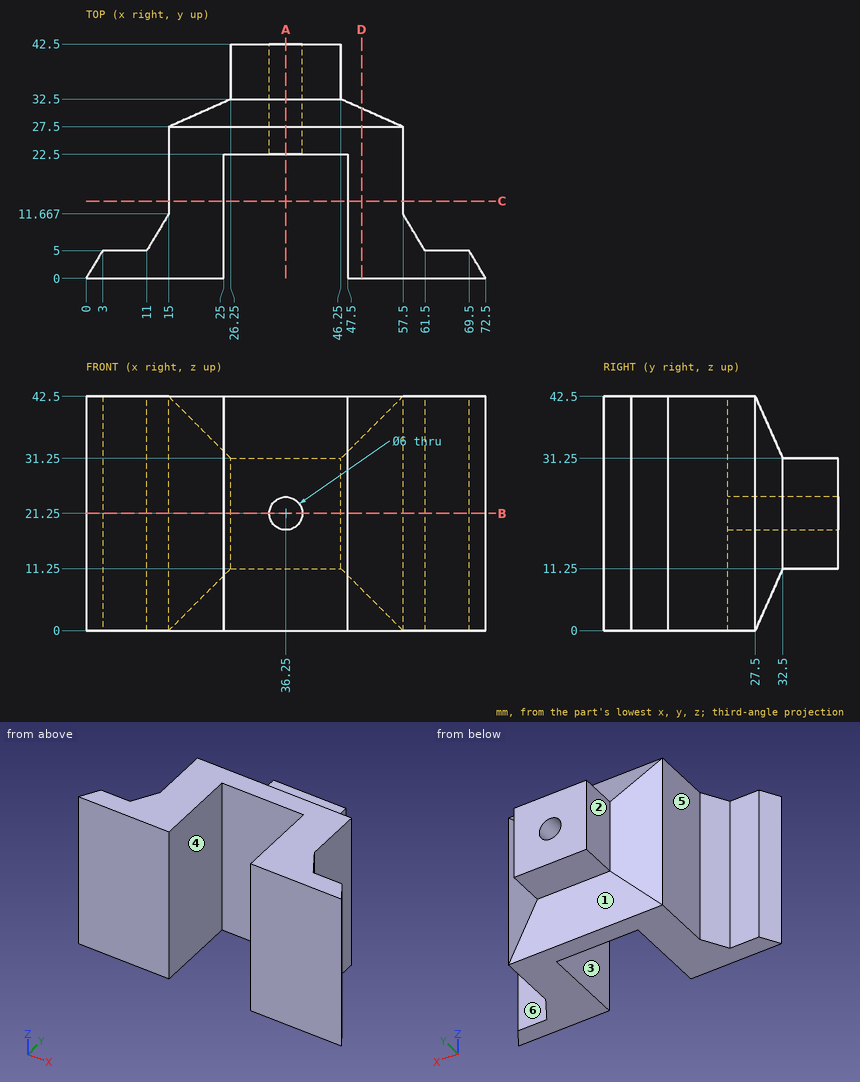
Geometry check sheet. Reference: drawing and pictorial views, mm from the part's lowest x, y, z. A direction names the side the tool comes from. Coordinates: 2 decimals unless noted, no trailing zeros. Loops run counter-clockwise (first coordinate to the right, second up) from the corner with the lowest first, then second, coordinate; pieces in that order, holes last.
1) Sectioned sample at C-C (y = 14). Record the boundary of the cut face in (x, z).
2) Sectioned sample at A-A (x = 36.25). Record the boundary of the cut face in (y, z).
3) Material ranges on probe 1 along Z at (x, y) = (36, 36); probe 2 along X at (y, z) = (21.5, 31); probe 3 along Y at (x, z) = (66, 18), recorded low to high.
4) Sectioned sample at D-D (x = 50). Record the boundary of the cut face in (y, z), and give its area (3 significant figures).
5) Gauge pin test, flat ends, axial feed: pin 1 (5.5 mm diameter, centred on x = 36.25, z = 21.25, fed in from -Y); pin 2 (5 mm diameter, centred on y = 15, z = 24, fed in from -X); pin 3 (1.5 mm diameter, centred on y = 31, z = 33.5, fed in from -X) (1 decimal); pin 4 (11 mm diameter, centred on y = 36, z = 20, fed in from +X). Record the tip position at first contact, or that the pin passes through.
6) Release check for a two-part mould opening along X. For the marked faces 1, 2 and 3 record: released by +X, released by -X, zero draft, split by the parting line, or undercut.
7) Access from +Z, -Z, +X, -X, +Y, -Y to the whole of each face (thin tool, end or side, straight path). Record for the marked faces 4, 5 and 6.
8) Sectioned sample at B-B (z = 21.25). Record the boundary of the cut face in (x, y).
Check sheet entries:
1. outline: (15, 0) - (25, 0) - (25, 42.5) - (15, 42.5) - close; (47.5, 0) - (57.5, 0) - (57.5, 42.5) - (47.5, 42.5) - close
2. outline: (22.5, 0) - (27.5, 0) - (32.5, 11.25) - (42.5, 11.25) - (42.5, 18.25) - (22.5, 18.25) - close; (22.5, 24.25) - (42.5, 24.25) - (42.5, 31.25) - (32.5, 31.25) - (27.5, 42.5) - (22.5, 42.5) - close
3. probe 1: z = 11.25 to 18.26, 24.24 to 31.25
3. probe 2: x = 15 to 25, 47.5 to 57.5
3. probe 3: y = 0 to 5
4. outline: (0, 0) - (27.5, 0) - (30.83, 7.5) - (30.83, 35) - (27.5, 42.5) - (0, 42.5) - close
4. area: 1,290 mm2
5. pin 1: passes through
5. pin 2: stops at x = 15
5. pin 3: stops at x = 21.2
5. pin 4: stops at x = 50.75
6. face 1: zero draft
6. face 2: released by -X
6. face 3: undercut
7. face 4: +Z, -Z, -Y
7. face 5: +Z, -Z, -X, +Y
7. face 6: +Z, -Z, +X, +Y
8. outline: (0, 0) - (25, 0) - (25, 22.5) - (33.25, 22.5) - (33.25, 42.5) - (26.25, 42.5) - (26.25, 32.5) - (15, 27.5) - (15, 11.67) - (11, 5) - (3, 5) - close; (39.25, 22.5) - (47.5, 22.5) - (47.5, 0) - (72.5, 0) - (69.5, 5) - (61.5, 5) - (57.5, 11.67) - (57.5, 27.5) - (46.25, 32.5) - (46.25, 42.5) - (39.25, 42.5) - close
